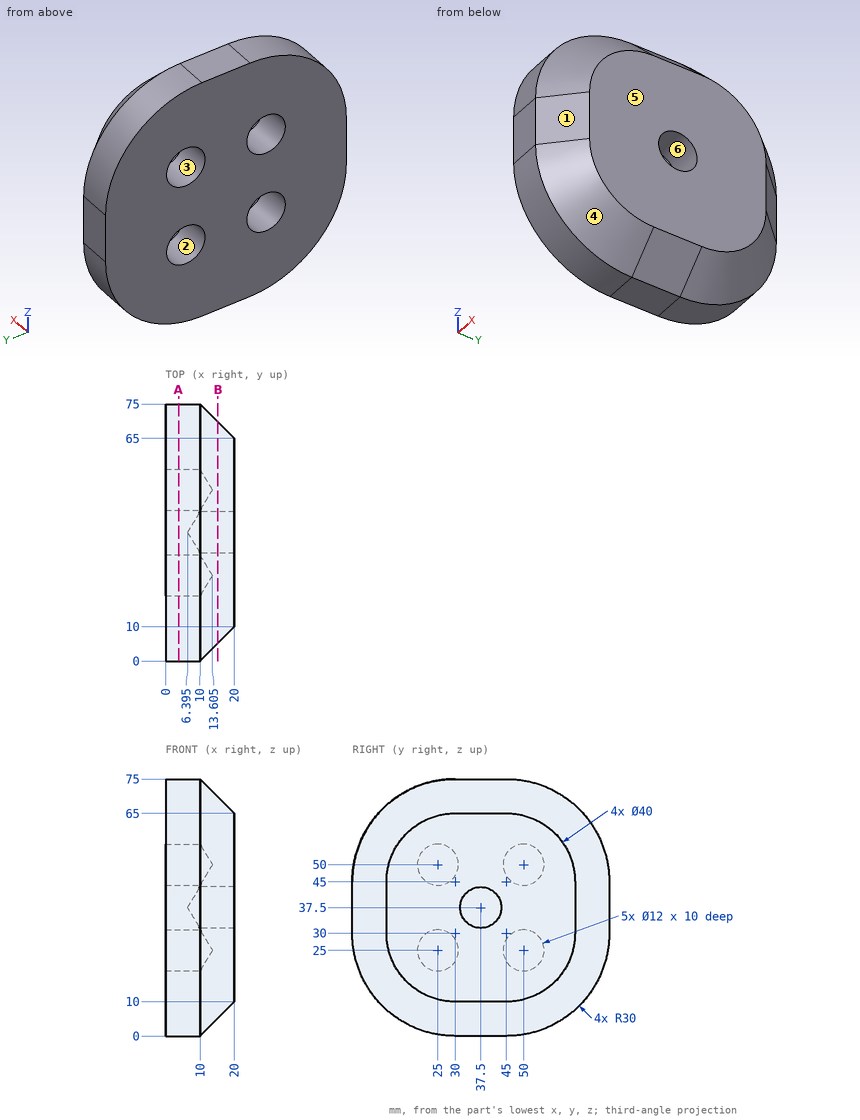
Geometry check sheet. Reference: drawing and pictorial views, mm from the part's lowest x, y, z. A direction names the side the tool comes from. Give positions to 0.01 mm unless a question says otherwise; leave off trailing zeros. Loops run counter-clockwise (first coordinate to the right, second up) from the corner with the lowest first, then second, coordinate; pieces in that order, holes last.
1. Section check A-A, the plane x = 3.75. Enter the section's corners in (y, z), then the cut area to 3 significant figures.
2. Set-up check for the marked faces 1 and 2: record each of +Z, -Z, +X, -X, +Y, -Y from which the full face is reachable in a straight line by a thin tool's end or side.
3. Thickness scan on line 1 (Z direction, x = 4.5, y = 25); line 2 (Z direction, x = 4.5, y = 24). Record the ranges inside material, lowest first.
4. Mould release check, pull along Z, two halves, no side actions. Record for the marked faces 3, 4, 5 and 6: released by +Z, released by -Z, zero draft, split by the parting line, or undercut.
5. Go/stop test with flat-tipped pins: pin 1 Ø4 at (x, z) = (7.5, 10.5) entering from -Y; pin 2 Ø1.5 at (x, y) = (17, 22) entering from -Z (1 decimal); pin 3 Ø3 at (x, y) = (2, 60.5) entering from -Z; pin 4 Ø5 at (x, y) = (2.5, 27.5) entering from +Z. Record where each tip stops, or that it passes through.
6. Section check B-B, the plane x = 15.25. Enter the section's corners in (y, z).
Geometry says:
1. outline: (0, 30) arc R30 ccw to (30, 0) - (45, 0) arc R30 ccw to (75, 30) - (75, 45) arc R30 ccw to (45, 75) - (30, 75) arc R30 ccw to (0, 45) - close; hole circle Ø12 at (25, 25); hole circle Ø12 at (25, 50); hole circle Ø12 at (50, 25); hole circle Ø12 at (50, 50)
1. area: 4,400 mm2
2. face 1: +Z, -Z, +X, -Y
2. face 2: -X
3. line 1: z = 0.42 to 19, 31 to 44, 56 to 74.58
3. line 2: z = 0.61 to 19.08, 30.92 to 44.08, 55.92 to 74.39
4. face 3: undercut
4. face 4: released by -Z
4. face 5: zero draft
4. face 6: undercut
5. pin 1: stops at y = 5.63
5. pin 2: stops at z = 7.6
5. pin 3: stops at z = 3.47
5. pin 4: stops at z = 75
6. outline: (5.25, 30) arc R24.75 ccw to (30, 5.25) - (45, 5.25) arc R24.75 ccw to (69.75, 30) - (69.75, 45) arc R24.75 ccw to (45, 69.75) - (30, 69.75) arc R24.75 ccw to (5.25, 45) - close; hole circle Ø12 at (37.5, 37.5)
